from build123d import *

# Parameters (mm, degrees)
F0_W          = 60
F0_H          = 14
F1_DEPTH      = 2
F2_W          = 60
F2_H          = 14
F3_DEPTH      = 1
F3_DEPTH_BACK = 1
F4_R          = 0.5
F6_DEPTH      = 25
F7_R          = 0.5


with BuildPart() as f1:
    # F0 (on Top) → F1 (new body)
    with BuildSketch(Plane.XY):
        with BuildLine():
            Line((31, 10), (-31, 10))
            ThreePointArc((-31, 10), (-32.4142135624, 9.4142135624), (-33, 8))
            Line((-33, 8), (-33, -8))
            ThreePointArc((-33, -8), (-32.4142135624, -9.4142135624), (-31, -10))
            Line((-31, -10), (31, -10))
            ThreePointArc((31, -10), (32.4142135624, -9.4142135624), (33, -8))
            Line((33, -8), (33, 8))
            ThreePointArc((33, 8), (32.4142135624, 9.4142135624), (31, 10))
        make_face()
        Rectangle(F0_W, F0_H, mode=Mode.SUBTRACT)
    extrude(amount=F1_DEPTH)

    # F2 (on face) → F3 (join, two sides)
    with BuildSketch(Plane.XY.offset(2)) as f3_sk:
        Rectangle(F2_W, F2_H)
    extrude(amount=F3_DEPTH)
    extrude(f3_sk.sketch, amount=-F3_DEPTH_BACK)

    # F4
    f4_edges = [f1.edges().sort_by_distance(p)[0] for p in [
        (-30, 7, 2.5),
        (-30, -7, 2.5),
        (30, -7, 2.5),
        (30, 7, 2.5),
    ]]
    fillet(f4_edges, radius=F4_R)

    # F5 (on Right) → F6 (cut, symmetric)
    with BuildSketch(Plane.YZ):
        with BuildLine():
            Line((-8.5, 2), (-9.5, 2))
            ThreePointArc((-9.5, 2), (-9, 1.5), (-8.5, 2))
        make_face()
        with BuildLine():
            ThreePointArc((8.5, 2), (9, 1.5), (9.5, 2))
            Line((9.5, 2), (8.5, 2))
        make_face()
    extrude(amount=F6_DEPTH, both=True, mode=Mode.SUBTRACT)

    # F7
    f7_edges = [f1.edges().sort_by_distance(p)[0] for p in [
        (30, -7, 0.5),
        (30, 7, 0.5),
        (-30, -7, 0.5),
        (-30, 7, 0.5),
    ]]
    fillet(f7_edges, radius=F7_R)


solid = f1.part
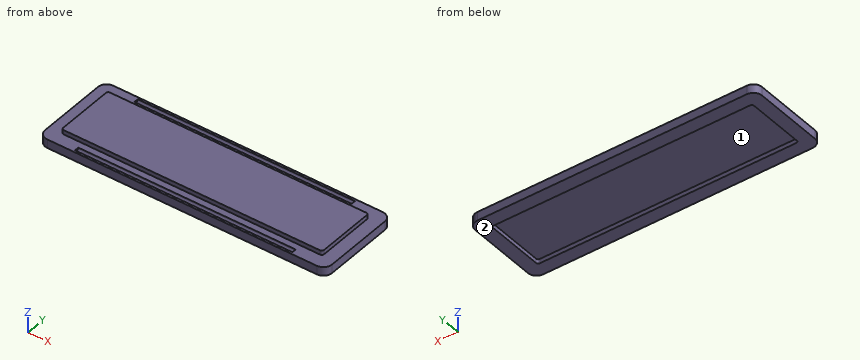
Verification items for the finished model (mm, model axes). Face numbers are marked on the shaded views. Coordinates: 2 decimals unless noted, no trailing zeros. Loops run counter-clockwise (first coordinate to the right, second up) from the corner with the lowest first, then second, coordinate; pieces in that order, holes last. Notation, with made-up numbers: (37, 46.5) -> (47, 46.5) arc R19 cw to (47, 53.5) -> close; hole circle Ø5 at (-32, -40). An arc over 180 degrees is marked (long way). Answer as a JSON object with one key per item and string values. Group by question number.
Item 1: Sectioned sample at A-A on x = -15. Record the boundary of the cut face in (y, z).
Item 2: Mould release check, pull along Y, two halves, no side actions. Record for the marked faces 1 and 2: +Y half, -Y half, draft (parallel to the pull), parting line (faces both ways), or undercut.
Item 3: Sectioned sample at B-B on y = 5. Record the boundary of the cut face in (x, z), plus the area to 3 significant figures.
Item 4: Depth check by flat-ended pin: pin 1 (0.8 mm diameter, centred on y = 2.5, z = 2.5, fed in from -X); pin 2 (0.6 mm diameter, centred on y = 9, z = 1.5, fed in from +X); pin 3 (6 mm diameter, centred on x = -4, y = 3, fed in from -Z). Enter the tip coordinate at first touch or a pass-through.
Item 5: Scan lines: probe 1 along Y at (x, z) = (-7, 1.9); probe 2 along Y at (x, z) = (7.5, 0.95); probe 3 along Y at (x, z) = (20, 1.7). Record each from-to range of solid material in increasing order.
Evaluation:
{
 "1": {"outline": "(-10, 0) -> (-7, 0) -> (-7, 1) -> (7, 1) -> (7, 0) -> (10, 0) -> (10, 2) -> (9.5, 2) arc R0.5 cw to (8.5, 2) -> (7, 2) -> (7, 3) -> (-7, 3) -> (-7, 2) -> (-8.5, 2) arc R0.5 cw to (-9.5, 2) -> (-10, 2) -> close"},
 "2": {"face 1": "undercut", "face 2": "draft"},
 "3": {"outline": "(-33, 0) -> (-30, 0) -> (-30, 1) -> (30, 1) -> (30, 0) -> (33, 0) -> (33, 2) -> (30, 2) -> (30, 3) -> (-30, 3) -> (-30, 2) -> (-33, 2) -> close", "area": "132 mm²"},
 "4": {"pin 1": "stops at x = -30", "pin 2": "stops at x = 32.87", "pin 3": "stops at z = 1"},
 "5": {"probe 1": "y = -10 to -9.49, -8.51 to 8.51, 9.49 to 10", "probe 2": "y = -10 to -7, 7 to 10", "probe 3": "y = -10 to -9.4, -8.6 to 8.6, 9.4 to 10"}
}
